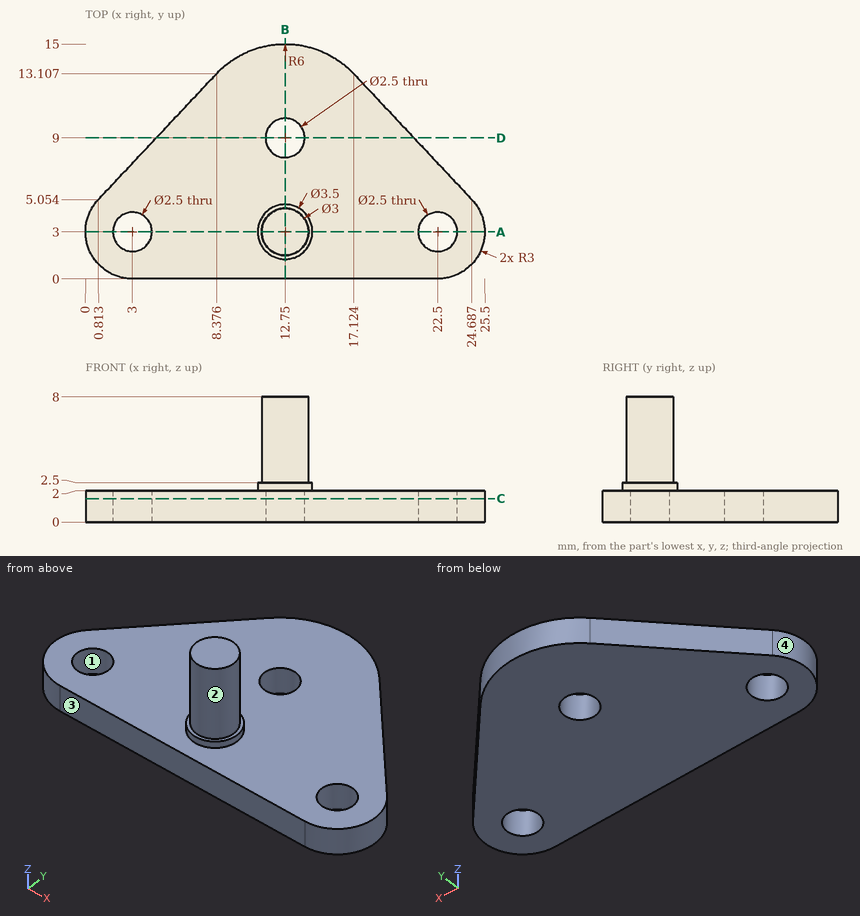
Source: three-view drawing plus pictorial views. Frame: mm from the lowest corner of the part. Give positions to 0.01 mm unless a question says otherwise; leave off trailing zeros. Write each loop counter-clockwise with the first axis right and the second up, starting at its lowest first coordinate (ties: lowest second). Pieces come first, ordered by that corner, then holes.
(1) Mould query, pull axis X, two halves, no side actions, for the marked faces 1, 2, 3 and 4. Classes: released by +X, released by -X, zero draft, split by the parting line, or undercut.
(2) Ray query, line 1 (Z direction, x = 9.75, y = 4.5); line 2 (Y direction, x = 16.5, z = 1) (1 decimal); line 3 (Y direction, x = 18.75, z = 1.5) (1 decimal). Return the intervals inside material, ascending.
(3) Cut plane D-D, the plane y = 9. Return loops of the section in (x, z), then the cut area to 3 significant figures.
(4) Cut plane C-C, the plane z = 1.5. Return loops of the section in (x, y).
(5) Cut plane B-B, the plane x = 12.75. Return loops of the section in (y, z).
(6) First-contact query: P1, Ø1.5, axis at y = 6, z = 1.5, coming from the +X side; P2, Ø1, axis at x = 17.5, y = 3.5, coming from the +Z side; P3, Ø1.5, axis at x = 14.5, z = 6, coming from the -Y side; P4, Ø2, axis at x = 22.5, y = 3, coming from the +Z side. Flat tips, straight axial feed; report the tip coordinate or a pass-through.
(7) Cut plane A-A, the plane y = 3. Return loops of the section in (x, z).
Values follow:
1. face 1: undercut
1. face 2: split by the parting line
1. face 3: zero draft
1. face 4: released by -X
2. line 1: z = 0 to 2
2. line 2: y = 0 to 13.7
2. line 3: y = 0 to 11.4
3. outline: (4.52, 0) - (11.5, 0) - (11.5, 2) - (4.52, 2) - close; (14, 0) - (20.98, 0) - (20.98, 2) - (14, 2) - close
3. area: 27.9 mm2
4. outline: (0.81, 5.05) arc R3 ccw to (3, 0) - (22.5, 0) arc R3 ccw to (24.69, 5.05) - (17.12, 13.11) arc R6 ccw to (8.38, 13.11) - close; hole circle Ø2.5 at (3, 3); hole circle Ø2.5 at (12.75, 9); hole circle Ø2.5 at (22.5, 3)
5. outline: (0, 0) - (7.75, 0) - (7.75, 2) - (4.75, 2) - (4.75, 2.5) - (4.5, 2.5) - (4.5, 8) - (1.5, 8) - (1.5, 2.5) - (1.25, 2.5) - (1.25, 2) - (0, 2) - close; (10.25, 0) - (15, 0) - (15, 2) - (10.25, 2) - close
6. P1: stops at x = 24.5
6. P2: stops at z = 2
6. P3: stops at y = 1.88
6. P4: passes through
7. outline: (0, 0) - (1.75, 0) - (1.75, 2) - (0, 2) - close; (4.25, 0) - (21.25, 0) - (21.25, 2) - (14.5, 2) - (14.5, 2.5) - (14.25, 2.5) - (14.25, 8) - (11.25, 8) - (11.25, 2.5) - (11, 2.5) - (11, 2) - (4.25, 2) - close; (23.75, 0) - (25.5, 0) - (25.5, 2) - (23.75, 2) - close
